```python
from build123d import *

# Parameters (mm, degrees)
BOSS_EXTRUDE1_DEPTH   = 9.7155
FILLET2_R             = 8.255
FILLET4_R             = 5.08
CROQUIS2_R            = 2.5
CORTAR_EXTRUIR2_DEPTH = 77.724


with BuildPart() as part:
    # Sketch1 → Boss-Extrude1 (new, symmetric)
    with BuildSketch(Plane.XY):
        with BuildLine():
            Line((-46.863, 0), (-46.863, 18.415))
            ThreePointArc((-46.863, 18.415), (-41.283384182, 31.885384182), (-27.813, 37.465))
            Line((-27.813, 37.465), (27.813, 37.465))
            ThreePointArc((27.813, 37.465), (41.283384182, 31.885384182), (46.863, 18.415))
            Line((46.863, 18.415), (46.863, 0))
            Line((46.863, 0), (63.5, 0))
            Line((63.5, 0), (63.5, 35.56))
            ThreePointArc((63.5, 35.56), (56.060512242, 53.520512242), (38.1, 60.96))
            Line((38.1, 60.96), (-38.1, 60.96))
            ThreePointArc((-38.1, 60.96), (-56.060512242, 53.520512242), (-63.5, 35.56))
            Line((-63.5, 35.56), (-63.5, 0))
            Line((-63.5, 0), (-46.863, 0))
        make_face()
    extrude(amount=BOSS_EXTRUDE1_DEPTH, both=True)

    # Fillet2
    fillet2_edges = [part.edges().sort_by_distance(p)[0] for p in [
        (56.060512242, 53.520512242, 9.7155),
        (-63.5, 17.78, -9.7155),
        (-46.863, 9.2075, -9.7155),
        (-41.283384182, 31.885384182, -9.7155),
        (0, 37.465, -9.7155),
        (41.283384182, 31.885384182, -9.7155),
        (63.5, 17.78, 9.7155),
        (46.863, 9.2075, -9.7155),
        (63.5, 17.78, -9.7155),
        (56.060512242, 53.520512242, -9.7155),
        (0, 60.96, -9.7155),
        (-56.060512242, 53.520512242, -9.7155),
        (46.863, 9.2075, 9.7155),
        (41.283384182, 31.885384182, 9.7155),
        (0, 37.465, 9.7155),
        (-41.283384182, 31.885384182, 9.7155),
        (-46.863, 9.2075, 9.7155),
        (-63.5, 17.78, 9.7155),
        (-56.060512242, 53.520512242, 9.7155),
        (0, 60.96, 9.7155),
    ]]
    fillet(fillet2_edges, radius=FILLET2_R)

    # Fillet4
    fillet4_edges = [part.edges().sort_by_distance(p)[0] for p in [
        (-55.1815, 0, 9.7155),
        (55.1815, 0, 9.7155),
        (-46.863, 0, 0),
        (-55.1815, 0, -9.7155),
        (-63.5, 0, 0),
        (-61.082166479, 0, 7.297666479),
        (-61.082166479, 0, -7.297666479),
        (-49.280833521, 0, -7.297666479),
        (-49.280833521, 0, 7.297666479),
        (46.863, 0, 0),
        (55.1815, 0, -9.7155),
        (63.5, 0, 0),
        (61.082166479, 0, 7.297666479),
        (61.082166479, 0, -7.297666479),
        (49.280833521, 0, -7.297666479),
        (49.280833521, 0, 7.297666479),
    ]]
    fillet(fillet4_edges, radius=FILLET4_R)

    # Croquis2 → Cortar-Extruir2 (cut, symmetric)
    with BuildSketch(Plane(origin=(0, 0, 0), x_dir=(0, 0, -1), z_dir=(1, 0, 0))):
        with Locations(Location((0, 5, 0), (0, 0, 1.833777999))):
            Circle(CROQUIS2_R)
    extrude(amount=CORTAR_EXTRUIR2_DEPTH, both=True, mode=Mode.SUBTRACT)


solid = part.part
```
Geometry: final body of the model. Coordinates: model frame, mm. A direction names the side the tool comes from. Round coordinates to 2 decimals unless told otherwise and drop trailing zeros. Order: outer loops, then holes, each group sorted by start corner. A loop starts at its lowest first (then second) coordinate and runs counter-clockwise, first axis right, second up. Notation, with made-up numbers: (25.5, 4) - (36.5, 4) arc R27 cw to (36.5, 33) - close; hole circle Ø1 at (23.5, 49.5). An arc over 180 degrees is marked (long way). Write item = value, one per line. Start each with the question number.
Q1. Cut plane B-B on z = 0. Return the cut outline in (x, y) (3 decimals).
Q2. Cut plane A-A on x = 1. Return the cut outline in (y, z) (1 decimal).
Q3. Access query for faces 1 (the cylindrical face through (49.16, 0.83, 0.02)), 2 (the cylindrical face through (49, 12, 7)), 3 (the cylindrical face through (-49, 12, -7)). Directions: +Z, -Z, +X, -X, +Y, -Y. A direction counts if a zero-diameter tool reaches every point of the face in a straight line with its end or side. Return the directions, or none.
Q4. Pull-direction query (X, two-part tool) for faces 4 (the cylindrical face through (49, 12, -7)), 5 (the cylindrical face through (61.2, 0.83, -0.02)), 6 (the flat face through (0, 48, 9.716)), 7 (the cylindrical face through (-61.133, 0.785, 0.02)); classes: +X half, -X half, draft (parallel to the pull), parting line (faces both ways), or undercut.
Q5. Ray query, line 1 (Z direction, x = 55, y = 5); line 2 (Z direction, x = -51.5, y = 5); line 3 (Y direction, x = 52.75, z = 0). Return the intervals inside material, ascending. Write a range as from..to.
Q6. Pin query (flat end, axial travel): pin 1 (1 mm diameter, centred on y = 35, z = -6, fed in from -X); pin 2 (5 mm diameter, centred on y = 39.5, z = 5, fed in from -X); pin 3 (1.5 mm diameter, centred on x = 12, z = 0, fed in from -Y) (3 decimals). Return the tip coordinate at first contact, or that it passes through.
Outcome:
q1.outline = (-63.5, 7.5) - (-46.863, 7.5) - (-46.863, 18.415) arc R19.05 cw to (-27.813, 37.465) - (27.813, 37.465) arc R19.05 cw to (46.863, 18.415) - (46.863, 7.5) - (63.5, 7.5) - (63.5, 35.56) arc R25.4 ccw to (38.1, 60.96) - (-38.1, 60.96) arc R25.4 ccw to (-63.5, 35.56) - close; (-62.796, 2.5) arc R5.08 ccw to (-58.42, 0) - (-51.943, 0) arc R5.08 ccw to (-47.567, 2.5) - close; (47.567, 2.5) arc R5.08 ccw to (51.943, 0) - (58.42, 0) arc R5.08 ccw to (62.796, 2.5) - close
q2.outline = (37.5, -1.5) arc R8.3 ccw to (45.7, -9.7) - (52.7, -9.7) arc R8.3 ccw to (61, -1.5) - (61, 1.5) arc R8.3 ccw to (52.7, 9.7) - (45.7, 9.7) arc R8.3 ccw to (37.5, 1.5) - close
q3.face_1 = +Z, -Z, -Y
q3.face_2 = +Z, -Y
q3.face_3 = -Z, -Y
q4.face_4 = undercut
q4.face_5 = +X half
q4.face_6 = draft
q4.face_7 = -X half
q5.line_1 = -9.71..-2.5, 2.5..9.71
q5.line_2 = -8.88..-2.5, 2.5..8.88
q5.line_3 = 0..2.5, 7.5..56.31
q6.pin_1 = -62.44
q6.pin_2 = -63.24
q6.pin_3 = 37.465
